```python
from build123d import *

# Parameters (mm, degrees)
F1_DEPTH = 400.05
F2_R     = 2.6162
F2_R_2   = 3.302
F3_DEPTH = 3.176
F4_R     = 2.6162
F5_DEPTH = 50.801


with BuildPart() as f1:
    # F0 (on Right) → F1 (new body)
    with BuildSketch(Plane.YZ):
        with BuildLine():
            Line((0, -44.45), (0, 0))
            Line((0, 0), (-3.175, 0))
            Line((-3.175, 0), (-3.175, -50.8))
            Line((-3.175, -50.8), (47.625, -50.8))
            Line((47.625, -50.8), (47.625, -47.625))
            Line((47.625, -47.625), (3.175, -47.625))
            ThreePointArc((3.175, -47.625), (0.929936, -46.695064), (0, -44.45))
        make_face()
    extrude(amount=-F1_DEPTH)

    # F2 (on face) → F3 (cut, through all)
    with BuildSketch(Plane(origin=(0, 0, 0), x_dir=(-1, 0, 0), z_dir=(0, 1, 0))):
        with Locations((9.525, -25.4)):
            Circle(F2_R)
        with Locations((390.525, -25.4)):
            Circle(F2_R)
        with Locations((177.0253, -41.305675)):
            Circle(F2_R_2)
        with Locations((223.0247, -41.305675)):
            Circle(F2_R_2)
        with Locations((177.0253, -28.300875)):
            Circle(F2_R_2)
        with Locations((223.0247, -28.300875)):
            Circle(F2_R_2)
        with Locations((159.439057, -34.803275)):
            Circle(F2_R)
        with Locations((240.5126, -34.803275)):
            Circle(F2_R)
        with Locations((249.5804, -7.9375)):
            Circle(F2_R)
        with Locations((150.4696, -7.9375)):
            Circle(F2_R)
    extrude(amount=-F3_DEPTH, mode=Mode.SUBTRACT)

    # F4 (on face) → F5 (cut, through all)
    with BuildSketch(Plane(origin=(0, 0, -50.8), x_dir=(1, 0, 0), z_dir=(0, 0, -1))):
        with Locations((-136.525, -9.525)):
            Circle(F4_R)
        with Locations((-136.525, -34.925)):
            Circle(F4_R)
        with Locations((-263.525, -9.525)):
            Circle(F4_R)
        with Locations((-263.525, -34.925)):
            Circle(F4_R)
    extrude(amount=-F5_DEPTH, mode=Mode.SUBTRACT)


solid = f1.part
```
The listing builds one solid part. Answer for the finished solid, in the listing's coordinates (mm). A direction names the side the tool comes from. Coordinates: 2 decimals unless noted, no trailing zeros. Write each loop counter-clockwise with the first axis right and the second up, starting at its lowest first coordinate (ties: lowest second). Pieces come first, ordered by that corner, then holes. Notation, with made-up numbers: (40.25, 83) - (82.25, 83) arc R24 ccw to (82.25, 93) - close; hole circle Ø6 at (29.25, 19.25). An arc over 180 degrees is marked (long way). Return JSON: item names as keys, results as strings. Group by question number.
1. Determine the mould class of faces 3 (the flat face through (-400.05, -0.5, -36.6)), 4 (the flat face through (-197, 26, -47.625)), 5 (the cylindrical face through (-222.31, -1.57, -44.53)), 6 (the flat face through (-197, 22, -50.8)) for opening direction Z: released by +Z, released by -Z, zero draft, split by the parting line, or undercut.
2. A cutting plane is placed at A-A, the plane x = -189.5. Determine the outline of the cut face in (y, z) (3 decimals).
3. Straight lines are drawn through the part: L1, parallel to Z at x = -308, y = 35 (3 decimals); L2, parallel to Y at x = -298, z = -8 (3 decimals). For each, find the intervals that lie inside material, in ascending order.
4. Given pin 1 (1 mm diameter, centred on x = -141.5, z = -10, fed in from +Y); pin 2 (10 mm diameter, centred on x = -355, y = 13.5, fed in from +Z) (3 decimals), each flat-ended and moving along its own axis, determine where each tip first touches the part or whether it passes through.
5. A cutting plane is placed at C-C, the plane y = 43. Determine the outline of the cut face in (x, z) (3 decimals), plus the area to 3 significant figures.
6. Which of the six approach directions +Z, -Z, +X, -X, +Y, -Y give full straight-line access (tool end or side, diameter ignored) to faces 1 (the cylindrical face through (-173.726, -1.565, -28.156)), 2 (the flat face through (-197, 0, -23))?
7. A cutting plane is placed at B-B, the plane z = -15. Determine the outline of the cut face in (x, y) (3 decimals), plus the area to 3 significant figures.
Ans:
{
 "1": {"face 3": "zero draft", "face 4": "released by +Z", "face 5": "undercut", "face 6": "released by -Z"},
 "2": {"outline": "(-3.175, -50.8) - (47.625, -50.8) - (47.625, -47.625) - (3.175, -47.625) arc R3.175 cw to (0, -44.45) - (0, 0) - (-3.175, 0) - close"},
 "3": {"L1": "-50.8 to -47.625", "L2": "-3.175 to 0"},
 "4": {"pin 1": "y = 0", "pin 2": "z = -47.625"},
 "5": {"outline": "(-400.05, -50.8) - (0, -50.8) - (0, -47.625) - (-400.05, -47.625) - close", "area": "1,270 mm²"},
 "6": {"face 1": "+Y, -Y", "face 2": "+Z, +X, -X, +Y"},
 "7": {"outline": "(-400.05, -3.175) - (0, -3.175) - (0, 0) - (-400.05, 0) - close", "area": "1,270 mm²"}
}
